Geometry: see drawing. Coordinates: mm, zero at the bounding-box minimum. A direction names the side the tool comes from. Give positions to 0.01 mm unless a question says otherwise; leave off trailing zeros. Order: outer loops, then holes, each group sorted by start corner. A loop starts at its lowest first (then second) coordinate and runs counter-clockwise, first axis right, second up. Notation, with made-up numbers: (-14, -35.5) - (4, -35.5) arc R10 cw to (4, -16.5) - close; hole circle Ø7 at (-33.75, -13.75). An arc over 180 degrees is marked (long way). Write item = value, one per line. Start each with the question number.
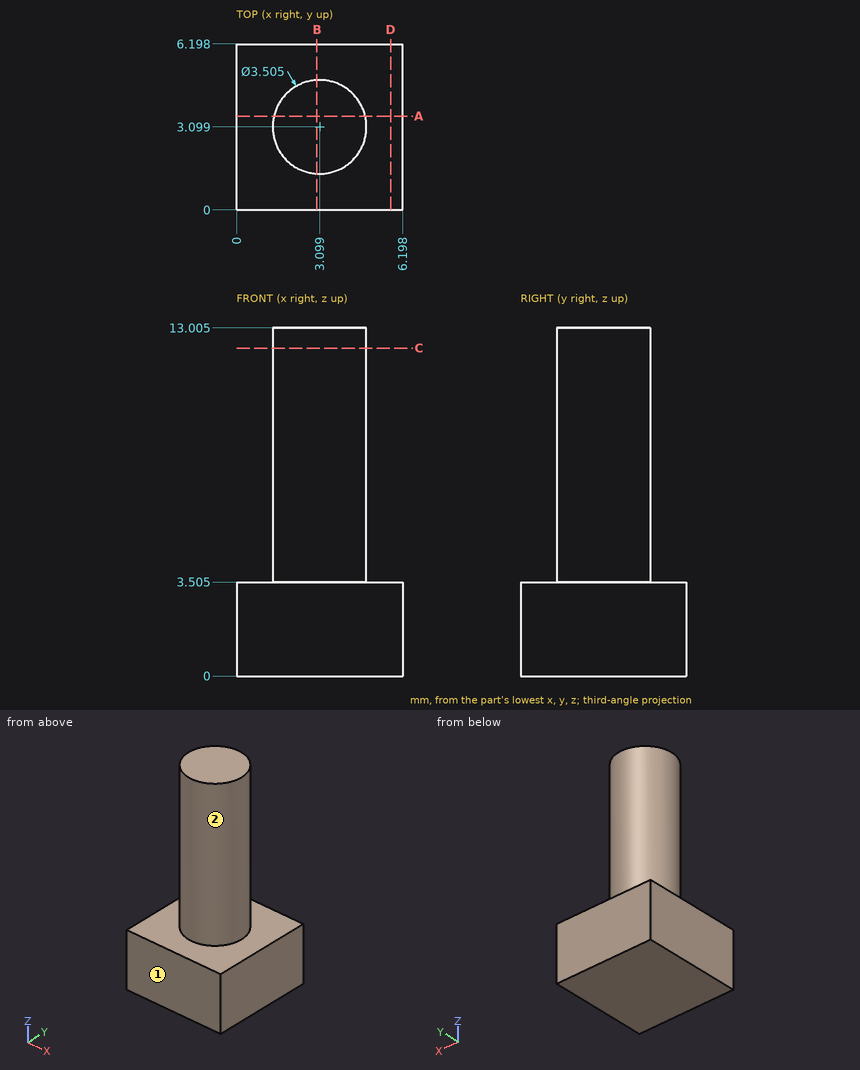
Q1. Material intervals for line 1 along Z through (x, y) = (4.75, 5.25) (1 decimal); line 2 along X through (y, z) = (3.25, 5.5) (1 decimal); line 3 along Y through (x, z) = (2, 11.5) (1 decimal), sorted ascending. Write a range as from..to.
Q2. Set-up query: the marked faces 1 and 2. Return all of +Z, -Z, +X, -X, +Y, -Y with unobstructed straight access to the full face (end or side cutting, diameter ignored); none if empty.
Q3. Section B-B, the plane x = 3. Return the cut outline in (y, z) (1 decimal).
Q4. Section D-D, the plane x = 5.75. Return the cut outline in (y, z) (1 decimal).
Q5. Section C-C, the plane z = 12.25. Return the cut outline in (x, y) (1 decimal).
Q6. Section A-A, the plane y = 3.5. Return the cut outline in (x, z) (1 decimal).
Q7. Contact query for flat-ended pins moving along their axis: pin 1 (3 mm diameter, centred on y = 1, z = 8, fed in from -X); pin 2 (2 mm diameter, centred on y = 5.5, z = 10.5, fed in from -X) (1 decimal); pin 3 (2 mm diameter, centred on y = 4, z = 11.5, fed in from -X). Output: stop coordinate, or through.
The answers:
q1.line_1 = 0..3.5
q1.line_2 = 1.4..4.8
q1.line_3 = 1.7..4.5
q2.face_1 = +Z, -Z, +X, -X, -Y
q2.face_2 = +Z
q3.outline = (0, 0) - (6.2, 0) - (6.2, 3.5) - (4.8, 3.5) - (4.8, 13) - (1.3, 13) - (1.3, 3.5) - (0, 3.5) - close
q4.outline = (0, 0) - (6.2, 0) - (6.2, 3.5) - (0, 3.5) - close
q5.outline = circle Ø3.5 at (3.1, 3.1)
q6.outline = (0, 0) - (6.2, 0) - (6.2, 3.5) - (4.8, 3.5) - (4.8, 13) - (1.4, 13) - (1.4, 3.5) - (0, 3.5) - close
q7.pin_1 = 1.45
q7.pin_2 = 2
q7.pin_3 = 1.35
